Can you work these out from the drawing? Everything is in mm from the part's minimum corner. Round coordinates to 2 decimals unless told otherwise and drop trailing zeros. Write each loop counter-clockwise with the first axis right and the second up, starting at its lowest first coordinate (ties: lowest second). Pieces come first, ordered by that corner, then holes.
Q1. If we section it at B-B (y = 68): Please give me the cut outline in (x, z), plus the area to 3 significant figures.
Q2. Please list where these lines run through material, in increasing order: line 1 along Y through (x, z) = (8.5, 4); line 2 along X through (y, z) = (14.5, 7.5); line 3 along Y through (x, z) = (96, 5.75).
Q3. If we section it at C-C (x = 88): Please give me the cut outline in (y, z).
Q4. If we section it at A-A (z = 8.75): Please give me the cut outline in (x, y), plus the area to 3 significant figures.
Q5. I'm going to push a flat-ended pin straight in: pin 1 Ø6 at (y, z) = (28.5, 6.5) entering from -X. Where does the tip first touch, or does it pass through?
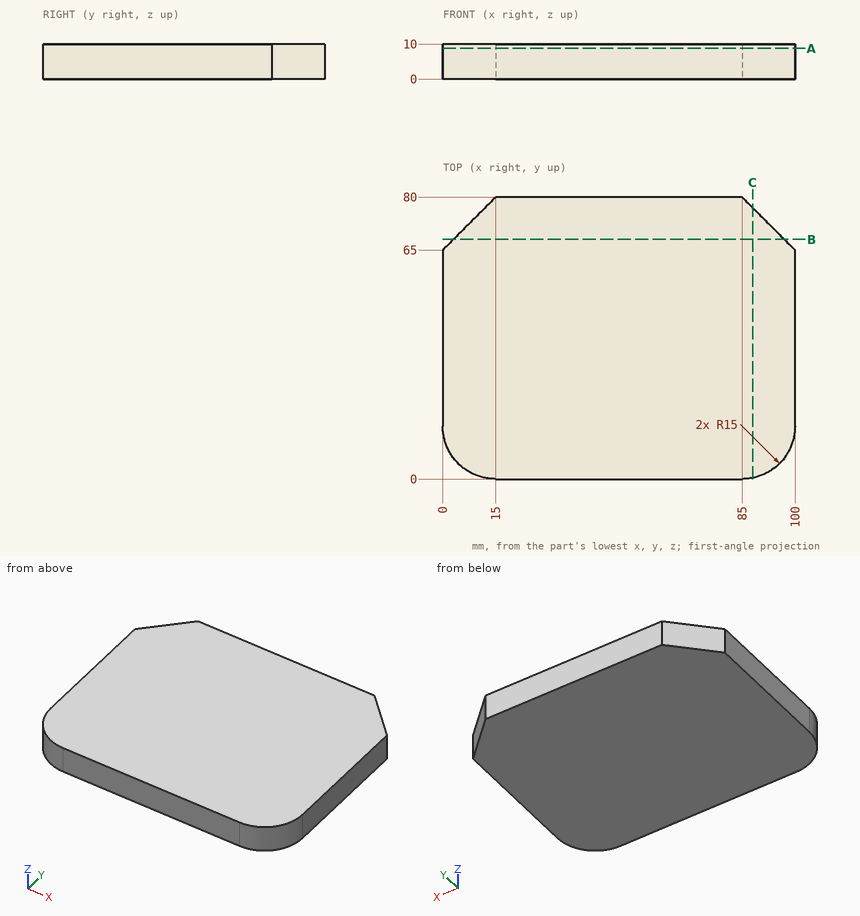
A:
1. outline: (3, 0) - (97, 0) - (97, 10) - (3, 10) - close
1. area: 940 mm2
2. line 1: y = 1.48 to 73.5
2. line 2: x = 0.01 to 99.99
2. line 3: y = 4.8 to 69
3. outline: (0.3, 0) - (77, 0) - (77, 10) - (0.3, 10) - close
4. outline: (0, 15) arc R15 ccw to (15, 0) - (85, 0) arc R15 ccw to (100, 15) - (100, 65) - (85, 80) - (15, 80) - (0, 65) - close
4. area: 7,680 mm2
5. pin 1: stops at x = 0
